```python
from build123d import *

# Parameters (mm, degrees)
CUT_EXTRUDE2_DEPTH = 1.925


with BuildPart() as part:
    # Sketch10 → Revolve3 (revolve)
    with BuildSketch(Plane(origin=(0, 0, 0), x_dir=(0, 0, -1), z_dir=(1, 0, 0)), mode=Mode.PRIVATE) as revolve3_sk:
        Polygon((27.15, 2.5), (27.75, 1.9), (27.75, 0), (2.75, 0), (2.75, 2.5), align=None)
    revolve(revolve3_sk.sketch.rotate(Axis((0, 0, 0), (0, 0, -1)), 90), axis=Axis((0, 0, 0), (0, 0, -1)))

    # Sketch7 → Revolve2 (revolve)
    with BuildSketch(Plane(origin=(0, 0, 0), x_dir=(0, 0, -1), z_dir=(1, 0, 0)), mode=Mode.PRIVATE) as revolve2_sk:
        with BuildLine():
            Line((2.3375, 4.75), (2.75, 4.75))
            Line((2.75, 4.75), (2.75, 0))
            Line((2.75, 0), (0, 0))
            Line((0, 0), (0, 2.5))
            ThreePointArc((0, 2.5), (0.991875183, 3.808753282), (2.3375, 4.75))
        make_face()
    revolve(revolve2_sk.sketch.rotate(Axis((0, 0, 0), (0, 0, -1)), 180), axis=Axis((0, 0, 0), (0, 0, -1)))

    # Sketch5 → Cut-Extrude2 (cut)
    with BuildSketch(Plane.XY):
        Polygon((1.5, -0.866025404), (1.5, 0.866025404), (0, 1.732050808), (-1.5, 0.866025404), (-1.5, -0.866025404), (0, -1.732050808), align=None)
    extrude(amount=-CUT_EXTRUDE2_DEPTH, mode=Mode.SUBTRACT)

    # Cut-Extrude3 cone 1 section (through the dimple's axis) → Cut-Extrude3 (revolve, cut)
    with BuildSketch(Plane(origin=(0, 0, 0), x_dir=(0, -1, 0), z_dir=(1, 0, 0))):
        Polygon((0, 0), (1.732050808, 0), (0, 1.732050808), align=None)
    revolve(axis=Axis((0, 0, 0), (0, 0, -1)), mode=Mode.SUBTRACT)


with BuildPart() as body_2:
    # Split1: read off the stored shape, not the designer's step
    # Split1: the piece on the far side of the plane
    add(part.part)
    split(bisect_by=Plane.XY.offset(-2.75), keep=Keep.BOTTOM)


with BuildPart() as part_1:
    add(part.part)

    # Split1
    split(bisect_by=Plane.XY.offset(-2.75), keep=Keep.TOP)


with BuildPart() as body_2_1:
    add(body_2.part)

    # Boss-Extrude1: read off the stored shape, not the designer's step
    # Boss-Extrude1: union part
    add(part_1.part)


solid = body_2_1.part
```
Source: CAD feature listing. Evaluate the final solid. Frame: model axes, mm. A direction names the side the tool comes from. Give positions to 0.01 mm unless a question says otherwise; leave off trailing zeros. Loops run counter-clockwise (first coordinate to the right, second up) from the corner with the lowest first, then second, coordinate; pieces in that order, holes last. Notation, with made-up numbers: (-15.5, -18.5) -> (38.5, -18.5) arc R25 ccw to (38.5, 6.5) -> close; hole circle Ø8 at (-16, -20.75). An arc over 180 degrees is marked (long way). Put each result on its own line as item: value. Start each with the question number.
1) Cut plane B-B (z = -14.25). Return loops of the section in (x, y).
2) Reachability of faces 4 (the face through (2, -1, 0)), 5 (the face through (2, -2, -2.75)), 6 (the face through (0.761, 1.293, -0.949)) from +Z, -Z, +X, -X, +Y, -Y: full face, straight path, thin tool, end or side. Return the list, or none.
3) Material intervals for probe 1 along X at (y, z) = (2, -4.75); probe 2 along Z at (x, y) = (0, -1) (3 decimals), sorted ascending.
4) Draft query along X for faces 1 (the face through (0, 0, -27.75)), 2 (the face through (0.8, 1.4, -0.12)), 3 (the face through (-2.5, -0.1, -15.1)). Return one class per face: released by +X, released by -X, zero draft, split by the parting line, or undercut.
5) Contact query for flat-ended pins moving along their axis: P1, Ø1.5, axis at y = 1, z = -8.5, coming from the +X side; P2, Ø0.5, axis at y = 0, z = -1, coming from the -X side; P3, Ø2, axis at x = 1, z = -7.5, coming from the +Y side. Output: stop coordinate, or through.
6) Cut plane C-C (x = -2.75). Return loops of the section in (y, z), then the cut area to 3 significant figures.
7) Cut plane D-D (y = 3.75). Return loops of the section in (x, z).
Results are:
1. outline: circle Ø5 at (0, 0)
2. face 4: +Z, +X, -X, +Y, -Y
2. face 5: -Z
2. face 6: +Z
3. probe 1: x = -1.5 to 1.5
3. probe 2: z = -27.75 to -1.925
4. face 1: zero draft
4. face 2: undercut
4. face 3: split by the parting line
5. P1: stops at x = 2.49
5. P2: stops at x = -4.04
5. P3: stops at y = 2.5
6. outline: (-3.87, -2.75) -> (3.87, -2.75) -> (3.87, -2.34) arc R4.51 ccw to (-3.87, -2.34) -> close
6. area: 15.2 mm2
7. outline: (-2.92, -2.75) -> (2.92, -2.75) -> (2.92, -2.34) arc R3.73 ccw to (-2.92, -2.34) -> close
